Check sheet for the modelled part. Datum: model origin and axes. Units: mm. A direction names the side the tool comes from. Give positions to 0.01 mm unless a question says otherwise; leave off trailing zeros. Write each loop counter-clockwise with the first axis right and the second up, starting at its lowest first coordinate (ties: lowest second). Pieces come first, ordered by that corner, then holes. Notation, with made-up numbers: (82, 69) -> (111, 69) arc R3 cw to (111, 74) -> close; hole circle Ø4 at (78, 38.25). An arc over 180 degrees is marked (long way). Answer as a JSON object with one key per item and string values.
from build123d import *

# Parameters (mm, degrees)
SKETCH1_W               = 26.5
SKETCH1_H               = 15.5
BOSS_EXTRUDE1_DEPTH     = 0.75
CUT_EXTRUDE1_START      = -1.5
CUT_EXTRUDE1_DEPTH      = 1.5
SKETCH3_R               = 16
CUT_EXTRUDE2_DEPTH      = 0.25
SKETCH5_R               = 13
CUT_EXTRUDE3_DEPTH      = 2.5
CUT_EXTRUDE9_DEPTH      = 2.5
SKETCH8_R               = 1.75
CUT_EXTRUDE6_DEPTH      = 2.5
SKETCH4_R               = 1.6
CUT_EXTRUDE7_DEPTH      = 1.75
CUT_EXTRUDE7_DEPTH_BACK = 1.75
CUT_EXTRUDE8_DEPTH      = 2.5
CUT_EXTRUDE10_DEPTH     = 2.5
CUT_EXTRUDE11_DEPTH     = 2.5
CHAMFER1_SIZE           = 0.2
CUT_EXTRUDE12_DEPTH     = 2.5
CIRPATTERN1_COUNT       = 2
CIRPATTERN1_ANGLE       = 45
MIRROR1_COPY_1_DEPTH    = 2.5


with BuildPart() as part:
    # Sketch1 → Boss-Extrude1 (new body, symmetric)
    with BuildSketch(Plane.XY):
        Rectangle(SKETCH1_W, SKETCH1_H)
    extrude(amount=BOSS_EXTRUDE1_DEPTH, both=True)

    # Sketch2 → Cut-Extrude1 (cut)
    with BuildSketch(Plane.XY.offset(0.75).offset(CUT_EXTRUDE1_START)):
        with BuildLine():
            Line((-13.25, 9.75), (-13.25, -1.486125371))
            ThreePointArc((-13.25, -1.486125371), (-1.032310159, 7.586384068), (13.25, 2.333005244))
            Line((13.25, 2.333005244), (13.25, 9.75))
            Line((13.25, 9.75), (-13.25, 9.75))
        make_face()
    extrude(amount=CUT_EXTRUDE1_DEPTH, mode=Mode.SUBTRACT)

    # Sketch3 → Cut-Extrude2 (cut, symmetric)
    with BuildSketch(Plane.XY):
        with Locations((1.25, -13.55)):
            Circle(SKETCH3_R)
    extrude(amount=CUT_EXTRUDE2_DEPTH, both=True, mode=Mode.SUBTRACT)

    # Sketch5 → Cut-Extrude3 (cut, through all)
    with BuildSketch(Plane.XY.offset(0.75)):
        with Locations((1.25, -13.55)):
            Circle(SKETCH5_R)
    extrude(amount=-CUT_EXTRUDE3_DEPTH, mode=Mode.SUBTRACT)

    # Sketch11 → Cut-Extrude9 (cut, through all)
    with BuildSketch(Plane.XY.offset(0.75)):
        with BuildLine():
            Line((11.255498488, -5.25), (13.25, -5.25))
            Line((13.25, -5.25), (13.25, -7.75))
            Line((13.25, -7.75), (12.884431658, -7.75))
            ThreePointArc((12.884431658, -7.75), (12.141930232, -6.453109426), (11.255498488, -5.25))
        make_face()
    extrude(amount=-CUT_EXTRUDE9_DEPTH, mode=Mode.SUBTRACT)

    # Sketch8 → Cut-Extrude6 (cut, through all)
    with BuildSketch(Plane.XY.offset(0.75)):
        with Locations((1.25, 5.45)):
            Circle(SKETCH8_R)
    extrude(amount=-CUT_EXTRUDE6_DEPTH, mode=Mode.SUBTRACT)

    # Sketch4 → Cut-Extrude7 (cut, two sides)
    with BuildSketch(Plane.XY) as cut_extrude7_sk:
        with Locations((1.721143205, -0.058223835)):
            Circle(SKETCH4_R)
        with Locations((6.307189011, -1.033017963)):
            Circle(SKETCH4_R)
        with Locations((10.283263186, -3.517544856)):
            Circle(SKETCH4_R)
        with Locations((-2.921729424, -0.71073703)):
            Circle(SKETCH4_R)
        with Locations((-7.061429917, -2.911854826)):
            Circle(SKETCH4_R)
        with Locations((-10.198649298, -6.396089933)):
            Circle(SKETCH4_R)
    extrude(amount=CUT_EXTRUDE7_DEPTH, mode=Mode.SUBTRACT)
    extrude(cut_extrude7_sk.sketch, amount=-CUT_EXTRUDE7_DEPTH_BACK, mode=Mode.SUBTRACT)

    # Sketch9 → Cut-Extrude8 (cut, through all)
    with BuildSketch(Plane.XY.offset(0.75)):
        with BuildLine():
            Line((-11.798649298, -6.396089933), (-11.798649298, -7.024324649))
            ThreePointArc((-11.798649298, -7.024324649), (-12.524324649, -7.75), (-13.25, -7.024324649))
            Line((-13.25, -7.024324649), (-13.25, -8.25))
            Line((-13.25, -8.25), (-11.05124975, -8.25))
            Line((-11.05124975, -8.25), (-11.05124975, -7.75))
            ThreePointArc((-11.05124975, -7.75), (-11.599392087, -7.169342569), (-11.798649298, -6.396089933))
        make_face()
    extrude(amount=-CUT_EXTRUDE8_DEPTH, mode=Mode.SUBTRACT)

    # Sketch12 → Cut-Extrude10 (cut, through all)
    with BuildSketch(Plane.XY.offset(0.75)):
        with BuildLine():
            Line((11.883263186, -3.517544856), (11.883263186, -4.566631593))
            ThreePointArc((11.883263186, -4.566631593), (12.566631593, -5.25), (13.25, -4.566631593))
            Line((13.25, -4.566631593), (13.25, -5.75))
            Line((13.25, -5.75), (11.255498488, -5.75))
            Line((11.255498488, -5.75), (11.255498488, -5.25))
            ThreePointArc((11.255498488, -5.25), (11.12789237, -5.098536084), (10.997993608, -4.949033739))
            ThreePointArc((10.997993608, -4.949033739), (11.644066014, -4.359100358), (11.883263186, -3.517544856))
        make_face()
    extrude(amount=-CUT_EXTRUDE10_DEPTH, mode=Mode.SUBTRACT)

    # Sketch13 → Cut-Extrude11 (cut, through all)
    with BuildSketch(Plane.XY.offset(0.75)):
        with BuildLine():
            Line((-8.661429917, -2.911854826), (-8.661429917, -5.042786286))
            ThreePointArc((-8.661429917, -5.042786286), (-8.818746964, -5.281977988), (-9.100687262, -5.232268912))
            ThreePointArc((-9.100687262, -5.232268912), (-8.836495341, -5.556723149), (-8.665455555, -5.938578244))
            ThreePointArc((-8.665455555, -5.938578244), (1.881828141, -1.065978484), (11.883263186, -6.978568343))
            Line((11.883263186, -6.978568343), (11.883263186, -3.517544856))
            ThreePointArc((11.883263186, -3.517544856), (10.883946092, -2.034581591), (9.134288128, -2.404056501))
            ThreePointArc((9.134288128, -2.404056501), (8.138950435, -2.52537475), (7.811663229, -1.577588737))
            ThreePointArc((7.811663229, -1.577588737), (6.906559561, 0.450476204), (4.846670181, -0.379653786))
            ThreePointArc((4.846670181, -0.379653786), (3.952851981, -0.83408119), (3.3211407, -0.055392485))
            ThreePointArc((3.3211407, -0.055392485), (1.7769824, 1.540801488), (0.125240729, 0.056210801))
            ThreePointArc((0.125240729, 0.056210801), (-0.559250312, -0.676515106), (-1.419191964, -0.160845059))
            ThreePointArc((-1.419191964, -0.160845059), (-3.200960568, 0.864708929), (-4.521729424, -0.71073703))
            Line((-4.521729424, -0.71073703), (-4.521729424, -1.460419063))
            ThreePointArc((-4.521729424, -1.460419063), (-5.006380866, -2.143921837), (-5.811741986, -1.912715158))
            ThreePointArc((-5.811741986, -1.912715158), (-7.590816029, -1.401970611), (-8.661429917, -2.911854826))
        make_face()
    extrude(amount=-CUT_EXTRUDE11_DEPTH, mode=Mode.SUBTRACT)

    # Chamfer1
    chamfer1_edges = [part.edges().sort_by_distance(p)[0] for p in [
        (-0.5, 5.45, -0.75),
    ]]
    chamfer(chamfer1_edges, length=CHAMFER1_SIZE)

    # Sketch14 → Cut-Extrude12 (cut)
    with BuildSketch(Plane.ZY.offset(-1.25)):
        Polygon((0.75, 5.85), (0.35, 5.45), (0.75, 5.05), align=None)
    cut_extrude12 = extrude(amount=CUT_EXTRUDE12_DEPTH, mode=Mode.SUBTRACT)

    # CirPattern1: Cut-Extrude12 ×2 about axis
    cirpattern1_axis = Axis((1.25, 5.45, 0), (0, 0, 1))
    for i in range(1, CIRPATTERN1_COUNT):
        add(cut_extrude12.rotate(cirpattern1_axis, i * CIRPATTERN1_ANGLE / (CIRPATTERN1_COUNT - 1)), mode=Mode.SUBTRACT)

    # Mirror1: Cut-Extrude12 across plane
    add(cut_extrude12.mirror(Plane.ZY.offset(-1.25)), mode=Mode.SUBTRACT)

    # Mirror1 copy 1 sketch → Mirror1 copy 1 (cut)
    with BuildSketch(Plane(origin=(-2.603731957, 1.596268043, 0), x_dir=(0, 0, 1), z_dir=(0.707106781, -0.707106781, 0))):
        Polygon((0.75, -5.85), (0.35, -5.45), (0.75, -5.05), align=None)
    extrude(amount=MIRROR1_COPY_1_DEPTH, mode=Mode.SUBTRACT)


solid = part.part
1. Scan lines: L1, parallel to Y at x = 1.25, z = -0.05; L2, parallel to X at y = -4.5, z = 0.35; L3, parallel to Z at x = -0.5, y = 4.75. Record each from-to range of solid material in increasing order. Write a range as [from, to].
Determined:
{"L1": "[2.45, 3.7], [7.2, 7.75]", "L2": "[-13.25, -8.66], [11.88, 13.25]", "L3": "[-0.68, 0.75]"}
2. Sectioned sample at A-A, the plane x = 1.25. Enter the section's corners in (y, z), plus the area to 3 significant figures.
Determined:
{"outline": "(1.47, -0.75) -> (3.5, -0.75) -> (3.7, -0.55) -> (3.7, 0.75) -> (1.47, 0.75) -> (1.47, 0.25) -> (2.45, 0.25) -> (2.45, -0.25) -> (1.47, -0.25) -> close; (7.2, -0.55) -> (7.4, -0.75) -> (7.75, -0.75) -> (7.75, 0.75) -> (7.2, 0.75) -> close", "area": "3.64 mm^2"}
3. Access from +Z, -Z, +X, -X, +Y, -Y to the whole of each face (thin tool, end or side, straight path). Record for faces 1 (the face through (-1.252, 7.553, -0.01)), 2 (the face through (-0.812, 2.317, 0.004)), 3 (the face through (-0.376, 4.111, 0.553)).
Determined:
{"face 1": "+Z, -Z, +Y", "face 2": "-Y", "face 3": "+Z"}
4. Sectioned sample at B-B, the plane x = 10.25. Enter the section's corners in (y, z).
Determined:
{"outline": "(-1.92, -0.75) -> (4.98, -0.75) -> (4.98, 0.75) -> (-1.92, 0.75) -> (-1.92, 0.25) -> (-0.32, 0.25) -> (-0.32, -0.25) -> (-1.92, -0.25) -> close"}
5. Go/stop test with flat-tipped pins: P1, Ø0.6, axis at y = -6.5, z = -0.5, coming from the +X side; P2, Ø1.5, axis at x = 1.5, y = 5.5, coming from the +Z side (3 decimals). Record where each tip stops, or that it passes through.
Determined:
{"P1": "x = -11.79", "P2": "through"}
6. Sectioned sample at C-C, the plane x = 5.75. Enter the section's corners in (y, z), plus the area to 3 significant figures.
Determined:
{"outline": "(0.47, -0.75) -> (7.1, -0.75) -> (7.1, 0.75) -> (0.47, 0.75) -> (0.47, 0.25) -> (1.8, 0.25) -> (1.8, -0.25) -> (0.47, -0.25) -> close", "area": "9.29 mm^2"}
7. Mould release check, pull along Z, two halves, no side actions. Record for faces 4 (the face through (-1, 0, -0.25)), 5 (the face through (2.876, 4.111, 0.553)), 6 (the face through (0, 2, -0.75)), 7 (the face through (-7.56, -1.39, -0.5)): released by +Z, released by -Z, zero draft, split by the parting line, or undercut.
Determined:
{"face 4": "undercut", "face 5": "released by +Z", "face 6": "released by -Z", "face 7": "zero draft"}
